The drawing under review shows one solid part. Ordinate dimensions are in mm from its lowest x, y, z. A direction names the side the tool comes from. Coordinates: 2 decimals unless noted, no trailing zeros. Write each loop counter-clockwise with the first axis right and the second up, starting at its lowest first coordinate (ties: lowest second). Pieces come first, ordered by that corner, then holes. Notation, with made-up numbers: (62.5, 28.5) -> (117.5, 28.5) arc R32 ccw to (117.5, 62.5) -> close; hole circle Ø5 at (27.25, 13.5). An arc over 180 degrees is marked (long way). One line per item, written item: value. Start each with the question number.
1) Add section D-D (z = 11.9). State the section outline as (x, y) points.
2) Mouldability with a two-part tool opening along Z and no side actions: class the marked faces 6, 7, 8 and 9 as released by +Z, released by -Z, zero draft, split by the parting line, or undercut.
3) For probe 1 along X at (y, z) = (1.1, 3.9); probe 2 along X at (y, z) = (0.9, 11.9); probe 3 along Y at (x, z) = (14.25, 5.75), list the stretches that pass through material, from the lowest coordinate up. Write a range as from..to.
4) Add section C-C (y = 4). State the section outline as (x, z) points, and give its area (3 significant figures).
5) For pin 1 Ø6 at (x, y) = (1.5, 3) entering from +Z; pin 2 Ø2.5 at (x, z) = (12, 12) entering from -Y, all flat-tipped, find the tip position at first contact; note any pin that passes through.
6) Add section B-B (x = 11.9). State the section outline as (y, z) points, and give its area (3 significant figures).
7) Add section A-A (z = 3.9). State the section outline as (x, y) points.
8) Machinability: for the marked faces 1, 2, 3, 4 and 5, which of the approach directions +Z, -Z, +X, -X, +Y, -Y give a long, thin tool a straight path to every point of the face, cutting with its end or side? Answer none if there is none.
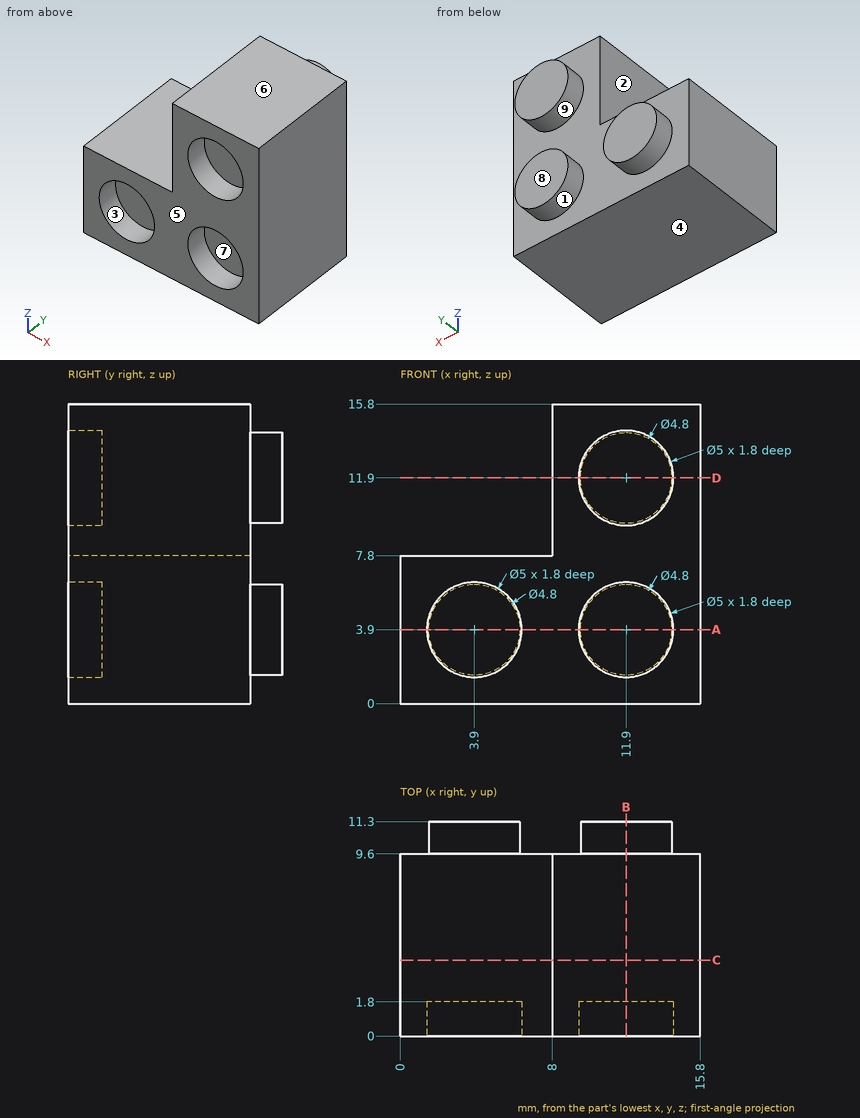
Numbers:
1. outline: (8, 0) -> (9.4, 0) -> (9.4, 1.8) -> (14.4, 1.8) -> (14.4, 0) -> (15.8, 0) -> (15.8, 9.6) -> (14.3, 9.6) -> (14.3, 11.3) -> (9.5, 11.3) -> (9.5, 9.6) -> (8, 9.6) -> close
2. face 6: released by +Z
2. face 7: undercut
2. face 8: zero draft
2. face 9: undercut
3. probe 1: 0..1.4, 6.4..9.4, 14.4..15.8
3. probe 2: 8..9.4, 14.4..15.8
3. probe 3: 0..9.6
4. outline: (0, 0) -> (15.8, 0) -> (15.8, 15.8) -> (8, 15.8) -> (8, 7.8) -> (0, 7.8) -> close
4. area: 186 mm²
5. pin 1: z = 7.8
5. pin 2: y = 1.8
6. outline: (0, 0) -> (9.6, 0) -> (9.6, 1.5) -> (11.3, 1.5) -> (11.3, 6.3) -> (9.6, 6.3) -> (9.6, 9.5) -> (11.3, 9.5) -> (11.3, 14.3) -> (9.6, 14.3) -> (9.6, 15.8) -> (0, 15.8) -> (0, 14.4) -> (1.8, 14.4) -> (1.8, 9.4) -> (0, 9.4) -> (0, 6.4) -> (1.8, 6.4) -> (1.8, 1.4) -> (0, 1.4) -> close
6. area: 150 mm²
7. outline: (0, 0) -> (1.4, 0) -> (1.4, 1.8) -> (6.4, 1.8) -> (6.4, 0) -> (9.4, 0) -> (9.4, 1.8) -> (14.4, 1.8) -> (14.4, 0) -> (15.8, 0) -> (15.8, 9.6) -> (14.3, 9.6) -> (14.3, 11.3) -> (9.5, 11.3) -> (9.5, 9.6) -> (6.3, 9.6) -> (6.3, 11.3) -> (1.5, 11.3) -> (1.5, 9.6) -> (0, 9.6) -> close
8. face 1: +Y
8. face 2: +Z, -X, +Y, -Y
8. face 3: -Y
8. face 4: -Z, +X, -X, +Y, -Y
8. face 5: +Z, -Z, +X, -X, -Y
